from build123d import *

# Parameters (mm, degrees)
SKETCH_1_R          = 2.25
EXTRUDE_1_DEPTH     = 9
SKETCH_2_R          = 4
CUT_EXTRUDE_1_DEPTH = 4
SKETCH_3_R          = 17
EXTRUDE_2_DEPTH     = 14
SKETCH_4_R          = 13
SKETCH_4_R_2        = 11
EXTRUDE_3_DEPTH     = 7.5
CUT_EXTRUDE_2_REACH = 44.571
SKETCH_5_R          = 5
CHAMFER_1_SIZE      = 1


with BuildPart() as part:
    # 草图1 → 凸台-拉伸1 (new body)
    with BuildSketch(Plane(origin=(0, 0, 0), x_dir=(1, 0, 0), z_dir=(0, 1, 0))):
        Polygon((0, 21), (15.769552622, 21), (21, 15.769552622), (21, 0), (21, -15.769552622), (15.769552622, -21), (0, -21), (-15.769552622, -21), (-21, -15.769552622), (-21, 0), (-21, 15.769552622), (-15.769552622, 21), align=None)
        with Locations(Location((14.849242405, 14.849242405, 0), (0, 0, 270))):
            Circle(SKETCH_1_R, mode=Mode.SUBTRACT)
        with Locations(Location((14.849242405, -14.849242405, 0), (0, 0, 270))):
            Circle(SKETCH_1_R, mode=Mode.SUBTRACT)
        with Locations(Location((-14.849242405, -14.849242405, 0), (0, 0, 270))):
            Circle(SKETCH_1_R, mode=Mode.SUBTRACT)
        with Locations(Location((-14.849242405, 14.849242405, 0), (0, 0, 270))):
            Circle(SKETCH_1_R, mode=Mode.SUBTRACT)
    extrude(amount=EXTRUDE_1_DEPTH)

    # 草图2 → 切除-拉伸1 (cut)
    with BuildSketch(Plane(origin=(0, 0, 0), x_dir=(1, 0, 0), z_dir=(0, 1, 0))):
        with Locations(Location((-14.849242405, 14.849242405, 0), (0, 0, 270))):
            Circle(SKETCH_2_R)
        with Locations(Location((14.849242405, 14.849242405, 0), (0, 0, 270))):
            Circle(SKETCH_2_R)
        with Locations(Location((14.849242405, -14.849242405, 0), (0, 0, 270))):
            Circle(SKETCH_2_R)
        with Locations(Location((-14.849242405, -14.849242405, 0), (0, 0, 270))):
            Circle(SKETCH_2_R)
    extrude(amount=CUT_EXTRUDE_1_DEPTH, mode=Mode.SUBTRACT)

    # 草图3 → 凸台-拉伸2 (add)
    with BuildSketch(Plane(origin=(0, 9, 0), x_dir=(1, 0, 0), z_dir=(0, 1, 0))):
        with Locations(Location((0, 0, 0), (0, 0, 270))):
            Circle(SKETCH_3_R)
    extrude(amount=EXTRUDE_2_DEPTH)

    # 草图4 → 凸台-拉伸3 (add)
    with BuildSketch(Plane.XZ):
        with Locations(Location((0, 0, 0), (0, 0, 270))):
            Circle(SKETCH_4_R)
        with Locations(Location((0, 0, 0), (0, 0, 270))):
            Circle(SKETCH_4_R_2, mode=Mode.SUBTRACT)
    extrude(amount=EXTRUDE_3_DEPTH)

    # 草图5 → 切除-拉伸2 (cut, up to next)
    with BuildSketch(Plane(origin=(0, 23, 0), x_dir=(1, 0, 0), z_dir=(0, 1, 0)), mode=Mode.PRIVATE) as cut_extrude_2_sk1:
        with Locations(Location((0, 0, 0), (0, 0, 270))):
            Circle(SKETCH_5_R)
    cut_extrude_2_tool1 = extrude(cut_extrude_2_sk1.sketch, amount=-CUT_EXTRUDE_2_REACH, mode=Mode.PRIVATE) & part.part
    add(cut_extrude_2_tool1.solids().sort_by_distance((0, 23, 0))[0], mode=Mode.SUBTRACT)

    # 倒角1
    chamfer_1_edges = [part.edges().sort_by_distance(p)[0] for p in [
        (0, 23, -17),
        (0, -7.5, 13),
    ]]
    chamfer(chamfer_1_edges, length=CHAMFER_1_SIZE)


solid = part.part
The model under review builds one solid part; all positions refer to its coordinate system, in mm. A direction names the side the tool comes from. Round coordinates to 2 decimals unless told otherwise and drop trailing zeros. Write each loop counter-clockwise with the first axis right and the second up, starting at its lowest first coordinate (ties: lowest second). Pieces come first, ordered by that corner, then holes. Notation, with made-up numbers: (-28.5, -34.75) - (4.5, -34.75) arc R23 ccw to (4.5, -11.75) - close; hole circle Ø7 at (42.5, 34.25). An arc over 180 degrees is marked (long way). One line per item, written item: value. Start each with the question number.
1. To check wall thickness, follow L1, parallel to Y at x = -5, z = 6; L2, parallel to Y at x = -6.5, z = -19; L3, parallel to X at y = 3.5, z = 17.5. State the ranges of each line that lie inside material, in increasing order. Write a range as from..to.
2. Consider section A-A on z = 0. Write out the cut boundary in (x, y).
3. The part is to be moulded in two halves that separate along X. For faces 3 (the face through (-17, 4, 17)), 4 (the face through (-14.673, 1.972, -18.845)), 5 (the face through (-18.42, 4.44, -18.35)), 6 (the face through (16.855, 15.409, -2.213)), say which applies: released by +X, released by -X, zero draft, split by the parting line, or undercut.
4. Consider section D-D on z = 14. State how many separate pieces and enclosed holes the cut face has, and give its area (3 significant figures).
5. Consider section C-C on y = 6. Write out the cut boundary in (x, z).
6. Clearance check with flat-ended pins moving along their axes: P1, Ø5, axis at x = -14.85, z = 14.85, coming from the -Y side; P2, Ø6.5, axis at x = -13, z = -15, coming from the -Y side; P3, Ø5, axis at x = 16.5, z = 9, coming from the +Y side; P4, Ø1.5, axis at x = -3.5, z = -2, coming from the +Y side. State where each tip first meets the part, or that it passes through.
7. Consider section B-B on x = 0. Write out the cut boundary in (y, z), and give its area (3 significant figures).
8. Machinability: for faces 1 (the face through (-17.283, 1.972, 11.675)), 2 (the face through (13.48, 6.465, 13.064)), which of the approach directions +Z, -Z, +X, -X, +Y, -Y give a long, thin tool a straight path to every point of the face, cutting with its end or side? Answer none if there is none.
Checks:
1. L1: y = 0..23
1. L2: y = 0..9
1. L3: x = -19.27..-17.84, -11.85..11.85, 17.84..19.27
2. outline: (-21, 0) - (-13, 0) - (-13, -6.5) - (-12, -7.5) - (-11, -7.5) - (-11, 0) - (-5, 0) - (-5, 23) - (-16, 23) - (-17, 22) - (-17, 9) - (-21, 9) - close; (5, 0) - (11, 0) - (11, -7.5) - (12, -7.5) - (13, -6.5) - (13, 0) - (21, 0) - (21, 9) - (17, 9) - (17, 22) - (16, 23) - (5, 23) - close
3. face 3: undercut
3. face 4: undercut
3. face 5: released by -X
3. face 6: split by the parting line
4. separate pieces: 3
4. enclosed holes: 0
4. area: 542 mm^2
5. outline: (-21, -15.77) - (-15.77, -21) - (15.77, -21) - (21, -15.77) - (21, 15.77) - (15.77, 21) - (-15.77, 21) - (-21, 15.77) - close; hole circle Ø4.5 at (-14.85, -14.85); hole circle Ø4.5 at (-14.85, 14.85); hole circle Ø10 at (0, 0); hole circle Ø4.5 at (14.85, -14.85); hole circle Ø4.5 at (14.85, 14.85)
6. P1: stops at y = 4
6. P2: stops at y = 0
6. P3: stops at y = 22.71
6. P4: passes through
7. outline: (-7.5, -12) - (-6.5, -13) - (0, -13) - (0, -21) - (9, -21) - (9, -17) - (22, -17) - (23, -16) - (23, -5) - (0, -5) - (0, -11) - (-7.5, -11) - close; (-7.5, 11) - (0, 11) - (0, 5) - (23, 5) - (23, 16) - (22, 17) - (9, 17) - (9, 21) - (0, 21) - (0, 13) - (-6.5, 13) - (-7.5, 12) - close
7. area: 652 mm^2
8. face 1: -Y
8. face 2: +Y, -Y
